Job drawing, mm, ordinate dimensions from the low corner. One solid piece. A direction names the side the tool comes from. Coordinates: 2 decimals unless noted, no trailing zeros. Loops run counter-clockwise (first coordinate to the right, second up) from the corner with the lowest first, then second, coordinate; pieces in that order, holes last. Notation, with made-up numbers: (44, 49) - (73, 49) arc R34 ccw to (73, 79) - close; hole circle Ø8 at (61.25, -2). An arc over 180 degrees is marked (long way). One line per question, with ' | ' between items. Start each with the question number.
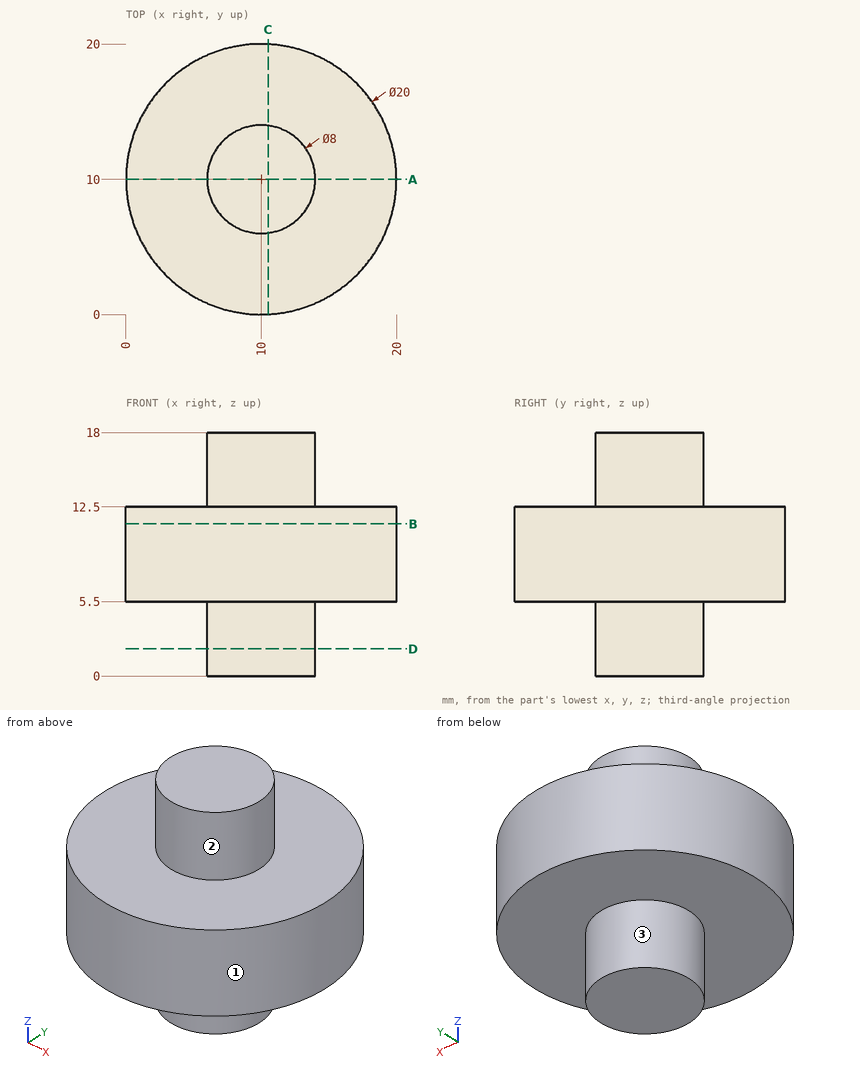
1) Band-saw the part on B-B on z = 11.25. List the corners of the cut face in (x, y), then the cut area to 3 significant figures.
2) Band-saw the part on C-C on x = 10.5. List the corners of the cut face in (y, z).
3) Band-saw the part on A-A on y = 10. List the corners of the cut face in (x, z).
4) Band-saw the part on D-D on z = 2. List the corners of the cut face in (x, y), then the cut area to 3 significant figures.
5) Wall check: line 1 along Z through (x, y) = (16.5, 12); line 2 along Y through (x, z) = (10.25, 8.75); line 3 along Y through (x, z) = (10, 13.5). Give the ranges that are in metal, low to high. Write a range as [from, to].
6) Tool access for the marked faces 1, 2 and 3: list every direction of +Z, -Z, +X, -X, +Y, -Y with a clear straight run to the whole face (end or side of a thin tool).
7) Pin check, flat tips, straight feed: pin 1 Ø5 at (x, z) = (5.5, 13) entering from +Y; pin 2 Ø10 at (x, y) = (16.5, 10) entering from +Z; pin 3 Ø3 at (y, z) = (15, 11.5) entering from +X; pin 4 Ø3 at (x, y) = (15, 16) entering from +Z. Stop position of each tip, or through.
Values found:
1) outline: circle Ø20 at (10, 10) | area: 314 mm²
2) outline: (0.01, 5.5) - (6.03, 5.5) - (6.03, 0) - (13.97, 0) - (13.97, 5.5) - (19.99, 5.5) - (19.99, 12.5) - (13.97, 12.5) - (13.97, 18) - (6.03, 18) - (6.03, 12.5) - (0.01, 12.5) - close
3) outline: (0, 5.5) - (6, 5.5) - (6, 0) - (14, 0) - (14, 5.5) - (20, 5.5) - (20, 12.5) - (14, 12.5) - (14, 18) - (6, 18) - (6, 12.5) - (0, 12.5) - close
4) outline: circle Ø8 at (10, 10) | area: 50.3 mm²
5) line 1: [5.5, 12.5] | line 2: [0, 20] | line 3: [6, 14]
6) face 1: +Z, -Z | face 2: +Z | face 3: -Z
7) pin 1: y = 19.79 | pin 2: z = 18 | pin 3: x = 19.37 | pin 4: z = 12.5
